Build history of the part. All positions in model axes, mm. A direction names the side the tool comes from. Coordinates: 2 decimals unless noted, no trailing zeros. Order: outer loops, then holes, each group sorted by start corner. A loop starts at its lowest first (then second) coordinate and runs counter-clockwise, first axis right, second up. Notation, with made-up numbers: M 83.5,14 L 110.5,14 A26 ccw 110.5,46 Z; hole C -35.5,-23.75 d4. An arc over 180 degrees is marked long. Use a Markdown table: item, result. Add a question column.
from build123d import *

# Parameters (mm, degrees)
EXTRUDE_1_DEPTH = 2
SKETCH_2_W      = 1.5
SKETCH_2_H      = 12
EXTRUDE_2_DEPTH = 1
SCALE_1_SCALE   = 1.6


with BuildPart() as part:
    # 草图1 → 凸台-拉伸1 (new body)
    with BuildSketch(Plane.XY):
        with BuildLine():
            Line((0, 7.5), (71.36690944, 7.5))
            Line((71.36690944, 7.5), (71.36690944, 6.01680195))
            Line((71.36690944, 6.01680195), (78.36690944, 6.01680195))
            Line((78.36690944, 6.01680195), (78.36690944, 7.5))
            Line((78.36690944, 7.5), (80.36690944, 7.5))
            Line((80.36690944, 7.5), (80.36690944, -7.5))
            Line((80.36690944, -7.5), (78.36690944, -7.5))
            Line((78.36690944, -7.5), (78.36690944, -6.01680195))
            Line((78.36690944, -6.01680195), (71.36690944, -6.01680195))
            Line((71.36690944, -6.01680195), (71.36690944, -7.5))
            Line((71.36690944, -7.5), (0, -7.5))
            ThreePointArc((0, -7.5), (-6.151670717, 0), (0, 7.5))
        make_face()
    extrude(amount=EXTRUDE_1_DEPTH)

    # 草图2 → 凸台-拉伸2 (add)
    with BuildSketch(Plane.XY.offset(2)):
        with Locations((3, 0)):
            Rectangle(SKETCH_2_W, SKETCH_2_H)
        with Locations((6, 0)):
            Rectangle(SKETCH_2_W, SKETCH_2_H)
        with Locations((9, 0)):
            Rectangle(SKETCH_2_W, SKETCH_2_H)
        with Locations((12, 0)):
            Rectangle(SKETCH_2_W, SKETCH_2_H)
        with Locations((15, 0)):
            Rectangle(SKETCH_2_W, SKETCH_2_H)
        with Locations((18, 0)):
            Rectangle(SKETCH_2_W, SKETCH_2_H)
        with Locations((21, 0)):
            Rectangle(SKETCH_2_W, SKETCH_2_H)
        with Locations((24, 0)):
            Rectangle(SKETCH_2_W, SKETCH_2_H)
        with Locations((27, 0)):
            Rectangle(SKETCH_2_W, SKETCH_2_H)
        with Locations((30, 0)):
            Rectangle(SKETCH_2_W, SKETCH_2_H)
        with Locations((33, 0)):
            Rectangle(SKETCH_2_W, SKETCH_2_H)
        with Locations((36, 0)):
            Rectangle(SKETCH_2_W, SKETCH_2_H)
        with Locations((39, 0)):
            Rectangle(SKETCH_2_W, SKETCH_2_H)
        with Locations((42, 0)):
            Rectangle(SKETCH_2_W, SKETCH_2_H)
        with Locations((45, 0)):
            Rectangle(SKETCH_2_W, SKETCH_2_H)
        with Locations((48, 0)):
            Rectangle(SKETCH_2_W, SKETCH_2_H)
        with Locations((51, 0)):
            Rectangle(SKETCH_2_W, SKETCH_2_H)
        with Locations((54, 0)):
            Rectangle(SKETCH_2_W, SKETCH_2_H)
        with Locations((57, 0)):
            Rectangle(SKETCH_2_W, SKETCH_2_H)
        with Locations((60, 0)):
            Rectangle(SKETCH_2_W, SKETCH_2_H)
        with Locations((63, 0)):
            Rectangle(SKETCH_2_W, SKETCH_2_H)
        with Locations((66, 0)):
            Rectangle(SKETCH_2_W, SKETCH_2_H)
        with Locations((69, 0)):
            Rectangle(SKETCH_2_W, SKETCH_2_H)
    extrude(amount=EXTRUDE_2_DEPTH)


with BuildPart() as part_1:
    # 缩放比例1: scaled about (37.07427317, 0, 1.212543803)
    add(part.part.scale(SCALE_1_SCALE).moved(Location((-22.244563902, 0, -0.727526282))))


solid = part_1.part
(1) Mould opens along X. For faces 4 (the flat face through (-13, 0, 4.072)), 5 (the flat face through (98, -9.627, 1)) say: released by +X, released by -X, zero draft, split by the parting line, or undercut.
(2) Slice it at A-A on x = -3. Give the cut face in (y, z).
(3) Which spindle directions (+Z, -Z, +X, -X, +Y, -Y) get a long thin tool onto all of the face, cutting with end or side? Do faces 1 (the flat face through (64, 0, 4.072)), 2 (the flat face through (91.942, -11, 1)), 3 (the flat face through (91.942, 11, 1)). Say none if no direction does.
(4) Slice it at B-B on z = 1. Give the cut face in (x, y).
(5) Drill centre lines: line 1 along Z through (x, y) = (-14, -3.25); line 2 along X through (y, z) = (-0.5, 0.15); line 3 along X through (y, z) = (-9.75, 0.2). Where is each one in solid material? Low to high. Write a range as from..to.
(6) Drop flat-ended pins along their axis: P1, Ø1.2, axis at y = 11, z = 0, coming from the -X side; P2, Ø0.5, axis at x = 1.5, z = 3.5, coming from the +Y side; P3, Ø0.5, axis at y = 4.5, z = 3.5, coming from the -X side. Give the stop position or say it passes through.
Solutions:
| question | item | result |
|---|---|---|
| 1 | face 4 | zero draft |
| 1 | face 5 | undercut |
| 2 | outline | M -12,-0.73 L 12,-0.73 L 12,2.47 L 9.6,2.47 L 9.6,4.07 L -9.6,4.07 L -9.6,2.47 L -12,2.47 Z |
| 3 | face 1 | +Z, +X, -X, +Y, -Y |
| 3 | face 2 | +Z, -Z, -Y |
| 3 | face 3 | +Z, -Z, +Y |
| 4 | outline | M -22.24,-12 L 91.94,-12 L 91.94,-9.63 L 103.14,-9.63 L 103.14,-12 L 106.34,-12 L 106.34,12 L 103.14,12 L 103.14,9.63 L 91.94,9.63 L 91.94,12 L -22.24,12 A12.24 ccw Z |
| 5 | line 1 | -0.73..2.47 |
| 5 | line 2 | -32.08..106.34 |
| 5 | line 3 | -27.24..91.94, 103.14..106.34 |
| 6 | P1 | x = -26.3 |
| 6 | P2 | y = 9.6 |
| 6 | P3 | x = -18.64 |
